from build123d import *

# Parameters (mm, degrees)
BOSS_EXTRU_1_DEPTH       = 270
ENL_V_MAT_EXTRU_4_DEPTH  = 26
ENL_V_MAT_EXTRU_5_DEPTH  = 20
ENL_V_MAT_EXTRU_6_DEPTH  = 42
ENL_V_MAT_EXTRU_7_DEPTH  = 19
ENL_V_MAT_EXTRU_8_DEPTH  = 10
ENL_V_MAT_EXTRU_9_DEPTH  = 10
ENL_V_MAT_EXTRU_10_DEPTH = 77
ENL_V_MAT_EXTRU_11_DEPTH = 10
ENL_V_MAT_EXTRU_12_DEPTH = 10
ENL_V_MAT_EXTRU_13_DEPTH = 37


with BuildPart() as part:
    # Esquisse1 → Boss.-Extru.1 (new body)
    with BuildSketch(Plane.XY):
        with BuildLine():
            Line((16.063962193, 30.398965806), (13.815004567, 31.398965806))
            Line((13.815004567, 31.398965806), (-11.613167833, 12.388079656))
            Line((-11.613167833, 12.388079656), (-8.463957616, 6.398855993))
            ThreePointArc((-8.463957616, 6.398855993), (-5.270411832, -5.520215773), (-5.985086805, -17.838991935))
            Line((-5.985086805, -17.838991935), (-5.985086805, -31.601034194))
            Line((-5.985086805, -31.601034194), (12.014913195, -31.601034194))
            ThreePointArc((12.014913195, -31.601034194), (7.480174869, -0.17266683), (16.063962193, 30.398965806))
        make_face()
    boss_extru_1 = extrude(amount=BOSS_EXTRU_1_DEPTH)

    # Esquisse3 → Enlèv. mat.-Extru.4 (cut)
    with BuildSketch(Plane.XY.offset(265)):
        with BuildLine():
            Line((-8.463957616, 6.398855993), (-11.613167833, 12.388079656))
            Line((-11.613167833, 12.388079656), (13.815004567, 31.398965806))
            ThreePointArc((13.815004567, 31.398965806), (4.532085849, 7.647429334), (3.665832045, -17.838991935))
            Line((3.665832045, -17.838991935), (-5.985086805, -17.838991935))
            ThreePointArc((-5.985086805, -17.838991935), (-5.270411832, -5.520215773), (-8.463957616, 6.398855993))
        make_face()
    enl_v_mat_extru_4 = extrude(amount=-ENL_V_MAT_EXTRU_4_DEPTH, mode=Mode.SUBTRACT)

    # Esquisse5 → Enlèv. mat.-Extru.5 (cut)
    with BuildSketch(Plane.XY.offset(239)):
        with BuildLine():
            Line((-8.463959076, 6.398857946), (-11.613169295, 12.388081611))
            Line((-11.613169295, 12.388081611), (13.815004567, 31.398965806))
            ThreePointArc((13.815004567, 31.398965806), (4.067679065, 5.247942268), (4.28050542, -22.659782317))
            Line((4.28050542, -22.659782317), (4.28050542, -27.25252086))
            Line((4.28050542, -27.25252086), (-5.985086805, -27.25252086))
            Line((-5.985086805, -27.25252086), (-5.985086805, -17.838991935))
            ThreePointArc((-5.985086805, -17.838991935), (-5.270412229, -5.520214661), (-8.463959076, 6.398857946))
        make_face()
    enl_v_mat_extru_5 = extrude(amount=-ENL_V_MAT_EXTRU_5_DEPTH, mode=Mode.SUBTRACT)

    # Esquisse6 → Enlèv. mat.-Extru.6 (cut)
    with BuildSketch(Plane.XY.offset(219)):
        with BuildLine():
            Line((-8.463957616, 6.398855993), (-11.613167833, 12.388079656))
            Line((-11.613167833, 12.388079656), (13.815004567, 31.398965806))
            ThreePointArc((13.815004567, 31.398965806), (10.20595229, 24.654084621), (7.296301708, 17.579297414))
            Line((7.296301708, 17.579297414), (-8.463957616, 6.398855993))
        make_face()
    enl_v_mat_extru_6 = extrude(amount=-ENL_V_MAT_EXTRU_6_DEPTH, mode=Mode.SUBTRACT)

    # Esquisse9 → Enlèv. mat.-Extru.7 (cut)
    with BuildSketch(Plane.XY.offset(177)):
        with BuildLine():
            Line((-8.521548111, 6.142905843), (-11.984807414, 12.729393608))
            Line((-11.984807414, 12.729393608), (14.702039036, 32.681300109))
            ThreePointArc((14.702039036, 32.681300109), (4.172070852, 5.87993715), (4.222916385, -22.91573442))
            Line((4.222916385, -22.91573442), (4.222916385, -27.508472963))
            Line((4.222916385, -27.508472963), (-6.04267584, -27.508472963))
            Line((-6.04267584, -27.508472963), (-6.04267584, -18.094944039))
            ThreePointArc((-6.04267584, -18.094944039), (-5.328001264, -5.776166764), (-8.521548111, 6.142905843))
        make_face()
    enl_v_mat_extru_7 = extrude(amount=-ENL_V_MAT_EXTRU_7_DEPTH, mode=Mode.SUBTRACT)

    # Esquisse10 → Enlèv. mat.-Extru.8 (cut)
    with BuildSketch(Plane.XY.offset(158)):
        with BuildLine():
            Line((-8.463957616, 6.398855993), (-11.613167833, 12.388079656))
            Line((-11.613167833, 12.388079656), (13.815004567, 31.398965806))
            ThreePointArc((13.815004567, 31.398965806), (4.532085849, 7.647429334), (3.665832045, -17.838991935))
            Line((3.665832045, -17.838991935), (-5.985086805, -17.838991935))
            ThreePointArc((-5.985086805, -17.838991935), (-5.270411832, -5.520215773), (-8.463957616, 6.398855993))
        make_face()
    enl_v_mat_extru_8 = extrude(amount=-ENL_V_MAT_EXTRU_8_DEPTH, mode=Mode.SUBTRACT)

    # Esquisse11 → Enlèv. mat.-Extru.9 (cut)
    with BuildSketch(Plane.XY.offset(144)):
        with BuildLine():
            Line((-8.463957616, 6.398855993), (-11.613167833, 12.388079656))
            Line((-11.613167833, 12.388079656), (13.815004567, 31.398965806))
            ThreePointArc((13.815004567, 31.398965806), (4.532085849, 7.647429334), (3.665832045, -17.838991935))
            Line((3.665832045, -17.838991935), (-5.985086805, -17.838991935))
            ThreePointArc((-5.985086805, -17.838991935), (-5.270411832, -5.520215773), (-8.463957616, 6.398855993))
        make_face()
    enl_v_mat_extru_9 = extrude(amount=-ENL_V_MAT_EXTRU_9_DEPTH, mode=Mode.SUBTRACT)

    # Esquisse12 → Enlèv. mat.-Extru.10 (cut)
    with BuildSketch(Plane.XY.offset(134)):
        with BuildLine():
            Line((-8.463959076, 6.398857946), (-11.613169295, 12.388081611))
            Line((-11.613169295, 12.388081611), (13.815004567, 31.398965806))
            ThreePointArc((13.815004567, 31.398965806), (4.067679065, 5.247942268), (4.28050542, -22.659782317))
            Line((4.28050542, -22.659782317), (4.28050542, -27.25252086))
            Line((4.28050542, -27.25252086), (-5.985086805, -27.25252086))
            Line((-5.985086805, -27.25252086), (-5.985086805, -17.838991935))
            ThreePointArc((-5.985086805, -17.838991935), (-5.270412229, -5.520214661), (-8.463959076, 6.398857946))
        make_face()
    enl_v_mat_extru_10 = extrude(amount=-ENL_V_MAT_EXTRU_10_DEPTH, mode=Mode.SUBTRACT)

    # Esquisse13 → Enlèv. mat.-Extru.11 (cut)
    with BuildSketch(Plane.XY.offset(57)):
        with BuildLine():
            Line((-8.463957616, 6.398855993), (-11.613167833, 12.388079656))
            Line((-11.613167833, 12.388079656), (13.815004567, 31.398965806))
            ThreePointArc((13.815004567, 31.398965806), (4.532085849, 7.647429334), (3.665832045, -17.838991935))
            Line((3.665832045, -17.838991935), (-5.985086805, -17.838991935))
            ThreePointArc((-5.985086805, -17.838991935), (-5.270411832, -5.520215773), (-8.463957616, 6.398855993))
        make_face()
    enl_v_mat_extru_11 = extrude(amount=-ENL_V_MAT_EXTRU_11_DEPTH, mode=Mode.SUBTRACT)

    # Esquisse14 → Enlèv. mat.-Extru.12 (cut)
    with BuildSketch(Plane.XY.offset(43)):
        with BuildLine():
            Line((-8.463957616, 6.398855993), (-11.613167833, 12.388079656))
            Line((-11.613167833, 12.388079656), (13.815004567, 31.398965806))
            ThreePointArc((13.815004567, 31.398965806), (4.532085849, 7.647429334), (3.665832045, -17.838991935))
            Line((3.665832045, -17.838991935), (-5.985086805, -17.838991935))
            ThreePointArc((-5.985086805, -17.838991935), (-5.270411832, -5.520215773), (-8.463957616, 6.398855993))
        make_face()
    enl_v_mat_extru_12 = extrude(amount=-ENL_V_MAT_EXTRU_12_DEPTH, mode=Mode.SUBTRACT)

    # Esquisse15 → Enlèv. mat.-Extru.13 (cut)
    with BuildSketch(Plane.XY.offset(33)):
        with BuildLine():
            Line((-8.463959076, 6.398857946), (-11.613169295, 12.388081611))
            Line((-11.613169295, 12.388081611), (13.815004567, 31.398965806))
            ThreePointArc((13.815004567, 31.398965806), (4.067679065, 5.247942268), (4.28050542, -22.659782317))
            Line((4.28050542, -22.659782317), (4.28050542, -27.25252086))
            Line((4.28050542, -27.25252086), (-5.985086805, -27.25252086))
            Line((-5.985086805, -27.25252086), (-5.985086805, -17.838991935))
            ThreePointArc((-5.985086805, -17.838991935), (-5.270412229, -5.520214661), (-8.463959076, 6.398857946))
        make_face()
    enl_v_mat_extru_13 = extrude(amount=-ENL_V_MAT_EXTRU_13_DEPTH, mode=Mode.SUBTRACT)

    # Symétrie1: Boss.-Extru.1, Enlèv. mat.-Extru.4, Enlèv. mat.-Extru.5, Enlèv. mat.-Extru.6, Enlèv. mat.-Extru.7, Enlèv. mat.-Extru.8, Enlèv. mat.-Extru.9, Enlèv. mat.-Extru.10, Enlèv. mat.-Extru.11, Enlèv. mat.-Extru.12, Enlèv. mat.-Extru.13 across plane
    add(boss_extru_1.mirror(Plane(origin=(0, 0, 0), x_dir=(1, 0, 0), z_dir=(0, 0, -1))))
    add(enl_v_mat_extru_4.mirror(Plane(origin=(0, 0, 0), x_dir=(1, 0, 0), z_dir=(0, 0, -1))), mode=Mode.SUBTRACT)
    add(enl_v_mat_extru_5.mirror(Plane(origin=(0, 0, 0), x_dir=(1, 0, 0), z_dir=(0, 0, -1))), mode=Mode.SUBTRACT)
    add(enl_v_mat_extru_6.mirror(Plane(origin=(0, 0, 0), x_dir=(1, 0, 0), z_dir=(0, 0, -1))), mode=Mode.SUBTRACT)
    add(enl_v_mat_extru_7.mirror(Plane(origin=(0, 0, 0), x_dir=(1, 0, 0), z_dir=(0, 0, -1))), mode=Mode.SUBTRACT)
    add(enl_v_mat_extru_8.mirror(Plane(origin=(0, 0, 0), x_dir=(1, 0, 0), z_dir=(0, 0, -1))), mode=Mode.SUBTRACT)
    add(enl_v_mat_extru_9.mirror(Plane(origin=(0, 0, 0), x_dir=(1, 0, 0), z_dir=(0, 0, -1))), mode=Mode.SUBTRACT)
    add(enl_v_mat_extru_10.mirror(Plane(origin=(0, 0, 0), x_dir=(1, 0, 0), z_dir=(0, 0, -1))), mode=Mode.SUBTRACT)
    add(enl_v_mat_extru_11.mirror(Plane(origin=(0, 0, 0), x_dir=(1, 0, 0), z_dir=(0, 0, -1))), mode=Mode.SUBTRACT)
    add(enl_v_mat_extru_12.mirror(Plane(origin=(0, 0, 0), x_dir=(1, 0, 0), z_dir=(0, 0, -1))), mode=Mode.SUBTRACT)
    add(enl_v_mat_extru_13.mirror(Plane(origin=(0, 0, 0), x_dir=(1, 0, 0), z_dir=(0, 0, -1))), mode=Mode.SUBTRACT)

    # Esquisse27 → Trou taraudé G1/162 (revolve, cut)
    with BuildSketch(Plane(origin=(3.014913195, -31.601034194, 247), x_dir=(0, 0, -1), z_dir=(1, 0, 0))):
        Polygon((0, 0), (0, 12), (3.3, 10.017159957), (3.3, 0), align=None)
    trou_taraud_g1_162 = revolve(axis=Axis((3.014913195, -37.951034194, 247), (0, 1, 0)), mode=Mode.SUBTRACT)

    # Esquisse28 → Trou taraudé G1/163 (revolve, cut)
    with BuildSketch(Plane(origin=(2.950249404, -31.601034194, 146), x_dir=(0, 0, -1), z_dir=(1, 0, 0))):
        Polygon((0, 0), (0, 12), (3.3, 10.017159957), (3.3, 0), align=None)
    trou_taraud_g1_163 = revolve(axis=Axis((2.950249404, -37.951034194, 146), (0, 1, 0)), mode=Mode.SUBTRACT)

    # Esquisse29 → Trou taraudé G1/164 (revolve, cut)
    with BuildSketch(Plane(origin=(3.014913195, -31.601034194, 45), x_dir=(0, 0, -1), z_dir=(1, 0, 0))):
        Polygon((0, 0), (0, 12), (3.3, 10.017159957), (3.3, 0), align=None)
    trou_taraud_g1_164 = revolve(axis=Axis((3.014913195, -37.951034194, 45), (0, 1, 0)), mode=Mode.SUBTRACT)

    # Symétrie2: Trou taraudé G1/162, Trou taraudé G1/163, Trou taraudé G1/164 across plane
    add(trou_taraud_g1_162.mirror(Plane(origin=(0, 0, 0), x_dir=(1, 0, 0), z_dir=(0, 0, -1))), mode=Mode.SUBTRACT)
    add(trou_taraud_g1_163.mirror(Plane(origin=(0, 0, 0), x_dir=(1, 0, 0), z_dir=(0, 0, -1))), mode=Mode.SUBTRACT)
    add(trou_taraud_g1_164.mirror(Plane(origin=(0, 0, 0), x_dir=(1, 0, 0), z_dir=(0, 0, -1))), mode=Mode.SUBTRACT)


solid = part.part
Model file for the job. Use its own axes, mm. Give positions to 0.01 mm unless a question says otherwise; leave off trailing zeros. Write each loop counter-clockwise with the first axis right and the second up, starting at its lowest first coordinate (ties: lowest second). Pieces come first, ordered by that corner, then holes. Notation, with made-up numbers: (-12.5, 78.5) -> (20.5, 78.5) arc R27 cw to (20.5, 95.5) -> close; hole circle Ø1 at (28, -13). An arc over 180 degrees is marked (long way). Write item = value, one per line.
(1) Probe line 1 along Z through (x, y) = (6, 18); line 2 along X through (y, z) = (-23.75, 146); line 3 along Y through (x, z) = (1.25, -140.5). List the from-to ranges inside material, lowest first.
Determined:
line_1 = -270 to -265, -148 to -144, -47 to -43, 43 to 47, 144 to 148, 265 to 270
line_2 = -5.99 to -0.35, 6.25 to 9.6
line_3 = -31.6 to -17.84
(2) Flat gauge pins, fed straight in: P1, Ø5, axis at y = -24.5, z = -100, coming from the -X side; P2, Ø6, axis at x = 3.01, z = 247, coming from the -Y side; P3, Ø1, axis at y = 19.5, z = 166.5, coming from the +X side. Where does each tip first touch, or does it go through?
Determined:
P1 = 4.16
P2 = -21.41
P3 = 11.57
(3) Slice it at A-A, the plane z = -93.5. Give the cut face in (x, y) (1 decimal).
Determined:
outline = (-6, -31.6) -> (12, -31.6) arc R76.7 cw to (16.1, 30.4) -> (13.8, 31.4) arc R77 ccw to (4.3, -22.7) -> (4.3, -27.3) -> (-6, -27.3) -> close
(4) Mould opens along Y. For faces 1 (the face through (1.279, 22.027, -145.972)), 2 (the face through (4.137, 5.635, 0.462)) say: released by +Y, released by -Y, zero draft, split by the parting line, or undercut.
Determined:
face_1 = released by +Y
face_2 = undercut
